Could you check a few things on this model? Use its own coordinates, in mm. A direction names the side the tool comes from. Round coordinates to 2 decimals unless told otherwise and drop trailing zeros. Order: outer loops, then holes, each group sorted by start corner. A loop starts at its lowest first (then second) coordinate and runs counter-clockwise, first axis right, second up.
```python
from build123d import *

# Parameters (mm, degrees)
SKETCH_1_W      = 24.75
SKETCH_1_H      = 32
EXTRUDE_1_DEPTH = 45
SKETCH_2_W      = 18.45
SKETCH_2_H      = 1.9
SKETCH_2_W_2    = 14
SKETCH_2_H_2    = 1.2
EXTRUDE_2_DEPTH = 28
SKETCH_4_R      = 9.6
SKETCH_4_R_2    = 1.5
EXTRUDE_3_DEPTH = 18.625


with BuildPart() as part:
    # 草图1 → 凸台-拉伸1 (new body)
    with BuildSketch(Plane.XY):
        with Locations((-0.370508982, -6.243263473)):
            Rectangle(SKETCH_1_W, SKETCH_1_H)
    extrude(amount=EXTRUDE_1_DEPTH)

    # 草图2 → 凸台-拉伸2 (add)
    with BuildSketch(Plane.XY.offset(45)):
        with Locations((-0.370508982, 10.706736527)):
            Rectangle(SKETCH_2_W, SKETCH_2_H)
        with Locations((-0.370508982, -22.843263473)):
            Rectangle(SKETCH_2_W_2, SKETCH_2_H_2)
    extrude(amount=-EXTRUDE_2_DEPTH)

    # 草图4 → 凸台-拉伸3 (add, symmetric)
    with BuildSketch(Plane(origin=(0, -6.243263473, 0), x_dir=(1, 0, 0), z_dir=(0, 1, 0))):
        with Locations(Location((-0.370508982, -10, 0), (0, 0, 226.816578204))):
            Circle(SKETCH_4_R)
        with Locations(Location((-0.370508982, -3, 0), (0, 0, 270))):
            Circle(SKETCH_4_R_2, mode=Mode.SUBTRACT)
        with Locations(Location((6.629491018, -10, 0), (0, 0, 270))):
            Circle(SKETCH_4_R_2, mode=Mode.SUBTRACT)
        with Locations((-0.370508982, -17)):
            Circle(SKETCH_4_R_2, mode=Mode.SUBTRACT)
        with Locations(Location((-7.370508982, -10, 0), (0, 0, 270))):
            Circle(SKETCH_4_R_2, mode=Mode.SUBTRACT)
    extrude(amount=EXTRUDE_3_DEPTH, both=True)


solid = part.part
```
Q1. Imagine slicing it at C-C, the plane z = 32.5. Please give me the cut outline in (x, y).
Q2. For faces 1 (the cylindrical face through (8.117, -23.574, 9.805)), 2 (the flat face through (0, 9.757, 3)), 3 (the flat face through (-12.746, -6, 22)), which set-ups out of +Z, -Z, +X, -X, +Y, -Y let a thin tool reach every point of the face, with its end or its side?
Q3. We'd pull the mould along X, two halves only. Please class faces 4 (the flat face through (-9.596, 11, 31)), 5 (the flat face through (0, -23.443, 31)), 6 (the flat face through (-7, 9.757, 10)), 7 (the cylindrical face through (-6.36, 11.05, 8.89)): released by +X, released by -X, zero draft, split by the parting line, or undercut.
Q4. Imagine slicing it at D-D, the plane z = 10. Please give me the cut outline in (x, y), then the cut area to 3 significant figures.
Q5. Imagine slicing it at B-B, the plane x = -3.5. Please give me the cut outline in (y, z).
Q6. I need wall thicknesses on L1, parallel to X at y = 10, z = 10; L2, parallel to X at y = -23, z = 3; L3, parallel to Y at x = 0.25, z = 4. Which ranges of each line are inside material? Lowest first, please.
Q7. Imagine slicing it at A-A, the plane z = 3. Please give me the cut outline in (x, y), then the cut area to 3 significant figures.
Q8. For P1, Ø1.5, axis at x = 6.5, z = 10.5, coming from the -Y side; P2, Ø5, axis at x = 6.63, z = 10, coming from the +Y side; P3, Ø0.6, axis at x = -0.5, y = 10.5, coming from the -Z side; P4, Ø8, axis at x = 0, z = 24, coming from the -Y side, each with a flat end and sliding along its axis, tell me the tip position at first contact or that it passes through.
Filled in:
1. outline: (-12.75, -22.24) - (-7.37, -22.24) - (-7.37, -23.44) - (6.63, -23.44) - (6.63, -22.24) - (12, -22.24) - (12, 9.76) - (8.85, 9.76) - (8.85, 11.66) - (-9.6, 11.66) - (-9.6, 9.76) - (-12.75, 9.76) - close
2. face 1: -Y
2. face 2: +Y
2. face 3: +Z, -Z, -X, +Y, -Y
3. face 4: released by -X
3. face 5: zero draft
3. face 6: undercut
3. face 7: undercut
4. outline: (-12.75, -22.24) - (-9.97, -22.24) - (-9.97, -24.87) - (-8.87, -24.87) - (-8.87, -22.24) - (-5.87, -22.24) - (-5.87, -24.87) - (5.13, -24.87) - (5.13, -22.24) - (8.13, -22.24) - (8.13, -24.87) - (9.23, -24.87) - (9.23, -22.24) - (12, -22.24) - (12, 9.76) - (9.23, 9.76) - (9.23, 12.38) - (8.13, 12.38) - (8.13, 9.76) - (5.13, 9.76) - (5.13, 12.38) - (-5.87, 12.38) - (-5.87, 9.76) - (-8.87, 9.76) - (-8.87, 12.38) - (-9.97, 12.38) - (-9.97, 9.76) - (-12.75, 9.76) - close
4. area: 861 mm2
5. outline: (-24.87, 0.92) - (-22.24, 0.92) - (-22.24, 0) - (9.76, 0) - (9.76, 0.92) - (12.38, 0.92) - (12.38, 19.08) - (11.66, 19.08) - (11.66, 45) - (-23.44, 45) - (-23.44, 19.08) - (-24.87, 19.08) - close
6. L1: x = -9.97 to -8.87, -5.87 to 5.13, 8.13 to 9.23
6. L2: x = -6.94 to -1.87, 1.13 to 6.2
6. L3: y = -22.24 to 9.76
7. outline: (-12.75, -22.24) - (-6.94, -22.24) - (-6.94, -24.87) - (-1.87, -24.87) - (-1.87, -22.24) - (1.13, -22.24) - (1.13, -24.87) - (6.2, -24.87) - (6.2, -22.24) - (12, -22.24) - (12, 9.76) - (6.2, 9.76) - (6.2, 12.38) - (1.13, 12.38) - (1.13, 9.76) - (-1.87, 9.76) - (-1.87, 12.38) - (-6.94, 12.38) - (-6.94, 9.76) - (-12.75, 9.76) - close
7. area: 845 mm2
8. P1: stops at y = -22.24
8. P2: stops at y = 12.38
8. P3: stops at z = 0.4
8. P4: stops at y = -23.44
